Could you check a few things on this drawing? It's one solid part, dimensions in mm from its lowest x, y, z. A direction names the side the tool comes from. Give positions to 0.01 mm unless a question says otherwise; leave off trailing zeros. Order: outer loops, then holes, each group sorted by start corner. A loop starts at its lowest first (then second) coordinate and runs counter-clockwise, first axis right, second up. Notation, with made-up numbers: (52.25, 46) - (107.25, 46) arc R18 cw to (107.25, 73) - close; hole circle Ø1 at (-29.5, 54). An arc over 180 degrees is marked (long way). One line per question, with ' | ' between items. Start each with the question number.
1. If we mould it in two halves opening along Y, with no side actions, what happens to the marked faces 3, 4 and 5? For each: released by +Y, released by -Y, zero draft, split by the parting line, or undercut.
2. For P1, Ø10, axis at x = 2, y = 7, coming from the +Z side (1 decimal); P2, Ø2, axis at x = 13, z = 19, coming from the +Y side (1 decimal); P3, Ø3, axis at x = 19.11, z = 11.11, coming from the +Y side, each with a flat end and sliding along its axis, tell me the tip position at first contact or that it passes through.
3. I need wall thicknesses on probe 1 along Y at (x, z) = (4.5, 6.5) (1 decimal); probe 2 along Y at (x, z) = (12, 20.5); probe 3 along X at (y, z) = (18.5, 13) (1 decimal). Which ranges of each line are inside material? Lowest first, please. Write a range as from..to.
4. Imagine slicing it at A-A (z = 8.5). Please give me the cut outline in (x, y) (1 decimal).
5. Which directions (+Z, -Z, +X, -X, +Y, -Y) give clear straight access to the entire face, cutting with the end or side of a thin tool? Please do the marked faces 1 and 2.
6. Imagine slicing it at B-B (x = 13.75). Please give me the cut outline in (y, z) (1 decimal).
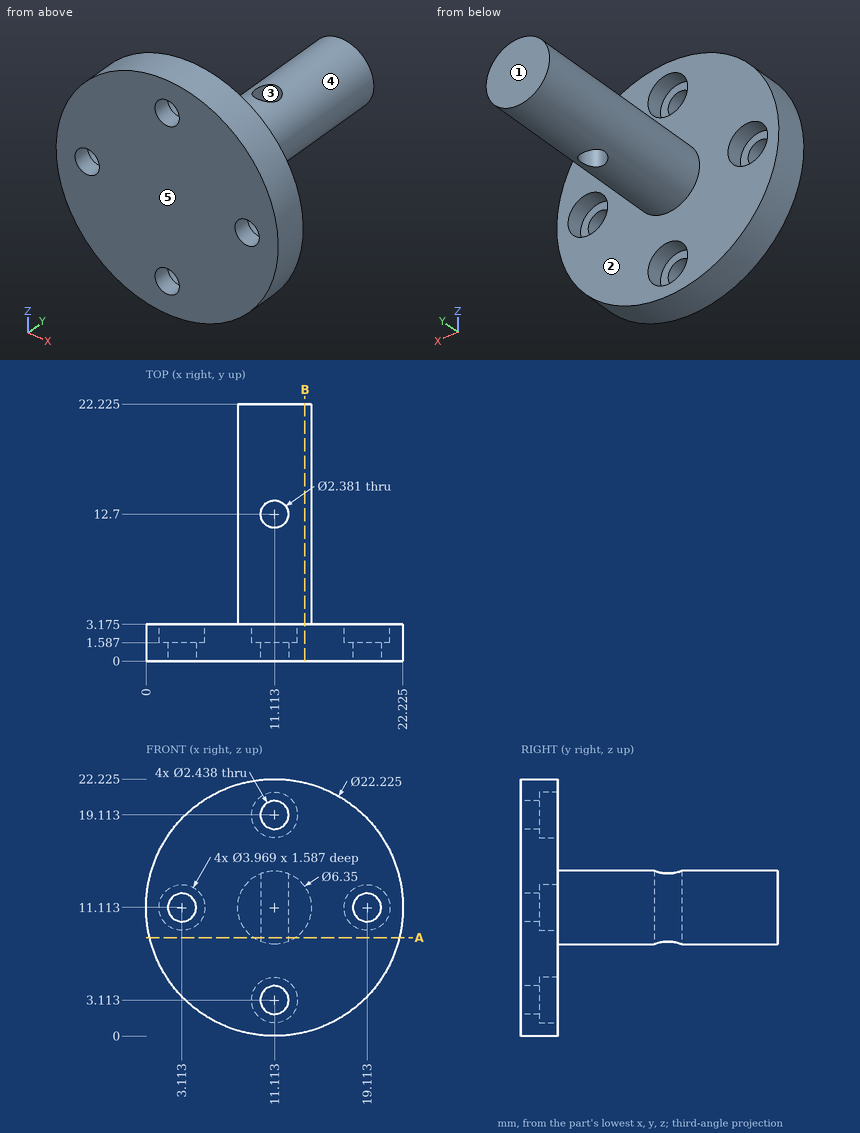
Results found:
1) face 3: undercut | face 4: zero draft | face 5: released by -Y
2) P1: stops at z = 20.5 | P2: stops at y = 3.2 | P3: stops at y = 1.59
3) probe 1: y = 0..3.2 | probe 2: y = 0..1.59 | probe 3: x = 8.6..13.7
4) outline: (0.3, 0) - (21.9, 0) - (21.9, 3.2) - (12.9, 3.2) - (12.9, 22.2) - (9.3, 22.2) - (9.3, 3.2) - (0.3, 3.2) - close; hole circle Ø2.4 at (11.1, 12.7)
5) face 1: +Z, -Z, +X, -X, +Y | face 2: +Y
6) outline: (0, 0.3) - (3.2, 0.3) - (3.2, 9.3) - (22.2, 9.3) - (22.2, 12.9) - (3.2, 12.9) - (3.2, 21.9) - (0, 21.9) - close
